from build123d import *

# Parameters (mm, degrees)
F0_R          = 12.5
F1_DEPTH      = 20
F1_DEPTH_BACK = 20
F3_DEPTH      = 40.001
F4_R          = 3
F5_DEPTH      = 25.001
F7_DEPTH      = 5


with BuildPart() as f1:
    # F0 (on Front) → F1 (new body, two sides)
    with BuildSketch(Plane.XZ) as f1_sk:
        with BuildLine():
            Line((49.364916731, 5), (19.364916731, 5))
            ThreePointArc((19.364916731, 5), (-20, 0), (19.364916731, -5))
            Line((19.364916731, -5), (49.364916731, -5))
            Line((49.364916731, -5), (49.364916731, 5))
        make_face()
        Circle(F0_R, mode=Mode.SUBTRACT)
    extrude(amount=F1_DEPTH)
    extrude(f1_sk.sketch, amount=-F1_DEPTH_BACK)

    # F2 (on face) → F3 (cut, through all)
    with BuildSketch(Plane.XZ.offset(20)):
        with BuildLine():
            Line((5.0842080384, 11.4193182205), (6.5077862892, 14.6167273223))
            ThreePointArc((6.5077862892, 14.6167273223), (4.6779472756, 15.3008760954), (2.7783708427, 15.7569240482))
            Line((2.7783708427, 15.7569240482), (2.1706022208, 12.3100969127))
            ThreePointArc((2.1706022208, 12.3100969127), (3.654646309, 11.9538094495), (5.0842080384, 11.4193182205))
        make_face()
        with BuildLine():
            Line((-3.8707503296, 15.5247316204), (-3.024023695, 12.1286965784))
            ThreePointArc((-3.024023695, 12.1286965784), (-1.5233667926, 12.4068268955), (0, 12.5))
            Line((0, 12.5), (0, 16))
            ThreePointArc((0, 16), (-1.9499094945, 15.8807384263), (-3.8707503296, 15.5247316204))
        make_face()
        with BuildLine():
            Line((-9.8505836052, 12.6081720577), (-7.6957684416, 9.8501344201))
            ThreePointArc((-7.6957684416, 9.8501344201), (-6.4379759364, 10.7145912588), (-5.0842080384, 11.4193182205))
            Line((-5.0842080384, 11.4193182205), (-6.5077862892, 14.6167273223))
            ThreePointArc((-6.5077862892, 14.6167273223), (-8.2406091986, 13.7146768112), (-9.8505836052, 12.6081720577))
        make_face()
        with BuildLine():
            Line((-14.1271614857, 7.5115450046), (-11.0368449107, 5.8683945348))
            ThreePointArc((-11.0368449107, 5.8683945348), (-10.2394005536, 7.1697054544), (-9.2893103185, 8.3641325795))
            Line((-9.2893103185, 8.3641325795), (-11.8903172076, 10.7060897017))
            ThreePointArc((-11.8903172076, 10.7060897017), (-13.1064327086, 9.1772229816), (-14.1271614857, 7.5115450046))
        make_face()
        with BuildLine():
            Line((-15.9610248042, 1.1161035799), (-12.4695506282, 0.8719559218))
            ThreePointArc((-12.4695506282, 0.8719559218), (-12.2703397931, 2.3851124422), (-11.8882064537, 3.8627124297))
            Line((-11.8882064537, 3.8627124297), (-15.2169042607, 4.94427191))
            ThreePointArc((-15.2169042607, 4.94427191), (-15.7060349352, 3.052943926), (-15.9610248042, 1.1161035799))
        make_face()
        with BuildLine():
            Line((-15.0350819326, -5.4723222932), (-11.7461577598, -4.2752517916))
            ThreePointArc((-11.7461577598, -4.2752517916), (-12.1796258098, -2.8118881793), (-12.4315236921, -1.3066057908))
            Line((-12.4315236921, -1.3066057908), (-15.9123503259, -1.6724554123))
            ThreePointArc((-15.9123503259, -1.6724554123), (-15.5899210366, -3.5992168695), (-15.0350819326, -5.4723222932))
        make_face()
        with BuildLine():
            Line((-11.5094368054, -11.1145339273), (-8.9917475042, -8.6832296307))
            ThreePointArc((-8.9917475042, -8.6832296307), (-9.9829438756, -7.5226877894), (-10.8253175473, -6.25))
            Line((-10.8253175473, -6.25), (-13.8564064606, -8))
            ThreePointArc((-13.8564064606, -8), (-12.7781681608, -9.6290403704), (-11.5094368054, -11.1145339273))
        make_face()
        with BuildLine():
            Line((-5.9937054947, -14.8349416731), (-4.6825824177, -11.5897981821))
            ThreePointArc((-4.6825824177, -11.5897981821), (-6.0601202531, -10.9327463392), (-7.3473156537, -10.1127124297))
            Line((-7.3473156537, -10.1127124297), (-9.4045640367, -12.94427191))
            ThreePointArc((-9.4045640367, -12.94427191), (-7.7569539239, -13.9939153142), (-5.9937054947, -14.8349416731))
        make_face()
        with BuildLine():
            Line((0.5583919472, -15.9902532323), (0.4362437088, -12.4923853377))
            ThreePointArc((0.4362437088, -12.4923853377), (-1.0894467843, -12.4524337261), (-2.5988961352, -12.2268450092))
            Line((-2.5988961352, -12.2268450092), (-3.3265870531, -15.6503616117))
            ThreePointArc((-3.3265870531, -15.6503616117), (-1.394491884, -15.9391151695), (0.5583919472, -15.9902532323))
        make_face()
        with BuildLine():
            Line((7.0139383486, -14.3807047408), (5.4796393349, -11.2349255787))
            ThreePointArc((5.4796393349, -11.2349255787), (4.0696019307, -11.818982195), (2.5988961352, -12.2268450092))
            Line((2.5988961352, -12.2268450092), (3.3265870531, -15.6503616117))
            ThreePointArc((3.3265870531, -15.6503616117), (5.2090904713, -15.1282972096), (7.0139383486, -14.3807047408))
        make_face()
        with BuildLine():
            Line((12.2567110899, -10.284601755), (9.575555539, -8.0348451211))
            ThreePointArc((9.575555539, -8.0348451211), (8.5249795008, -9.1419212702), (7.3473156537, -10.1127124297))
            Line((7.3473156537, -10.1127124297), (9.4045640367, -12.94427191))
            ThreePointArc((9.4045640367, -12.94427191), (10.911973761, -11.7016592259), (12.2567110899, -10.284601755))
        make_face()
        with BuildLine():
            Line((15.380187135, -4.4101976931), (12.0157711992, -3.4454669477))
            ThreePointArc((12.0157711992, -3.4454669477), (11.5063106682, -4.8841391061), (10.8253175473, -6.25))
            Line((10.8253175473, -6.25), (13.8564064606, -8))
            ThreePointArc((13.8564064606, -8), (14.7280776552, -6.2516980558), (15.380187135, -4.4101976931))
        make_face()
        with BuildLine():
            Line((15.8442890999, 2.2267696154), (12.3783508593, 1.739663762))
            ThreePointArc((12.3783508593, 1.739663762), (12.4980961895, 0.2181550805), (12.4315236921, -1.3066057908))
            Line((12.4315236921, -1.3066057908), (15.9123503259, -1.6724554123))
            ThreePointArc((15.9123503259, -1.6724554123), (15.9975631225, 0.279238503), (15.8442890999, 2.2267696154))
        make_face()
        with BuildLine():
            Line((13.5687695385, 8.4787082277), (10.600601202, 6.6239908029))
            ThreePointArc((10.600601202, 6.6239908029), (11.328847338, 5.2827282718), (11.8882064537, 3.8627124297))
            Line((11.8882064537, 3.8627124297), (15.2169042607, 4.94427191))
            ThreePointArc((15.2169042607, 4.94427191), (14.5009245926, 6.7618921879), (13.5687695385, 8.4787082277))
        make_face()
        with BuildLine():
            Line((8.9470864555, 13.2646011609), (6.9899112934, 10.3629696569))
            ThreePointArc((6.9899112934, 10.3629696569), (8.2007378624, 9.4338697528), (9.2893103185, 8.3641325795))
            Line((9.2893103185, 8.3641325795), (11.8903172076, 10.7060897017))
            ThreePointArc((11.8903172076, 10.7060897017), (10.4969444638, 12.0753532836), (8.9470864555, 13.2646011609))
        make_face()
    extrude(amount=-F3_DEPTH, mode=Mode.SUBTRACT)

    # F4 (on face) → F5 (cut, through all)
    with BuildSketch(Plane.XY.offset(5)):
        with Locations((26, 14)):
            Circle(F4_R)
        with Locations((42, 14)):
            Circle(F4_R)
        with Locations((26, -14)):
            Circle(F4_R)
        with Locations((42, -14)):
            Circle(F4_R)
    extrude(amount=-F5_DEPTH, mode=Mode.SUBTRACT)

    # F6 (on face) → F7 (cut)
    with BuildSketch(Plane(origin=(0, 0, -5), x_dir=(1, 0, 0), z_dir=(0, 0, -1))):
        Polygon((31.7735026919, 14), (28.8867513459, 19), (23.1132486541, 19), (20.2264973081, 14), (23.1132486541, 9), (28.8867513459, 9), align=None)
        Polygon((39.1132486541, 9), (44.8867513459, 9), (47.7735026919, 14), (44.8867513459, 19), (39.1132486541, 19), (36.2264973081, 14), align=None)
        Polygon((39.1132486541, -9), (36.2264973081, -14), (39.1132486541, -19), (44.8867513459, -19), (47.7735026919, -14), (44.8867513459, -9), align=None)
        Polygon((20.2264973081, -14), (23.1132486541, -19), (28.8867513459, -19), (31.7735026919, -14), (28.8867513459, -9), (23.1132486541, -9), align=None)
    extrude(amount=-F7_DEPTH, mode=Mode.SUBTRACT)


solid = f1.part
Geometry check sheet. Reference: the model listing, model coordinates, mm. A direction names the side the tool comes from. Round coordinates to 2 decimals unless told otherwise and drop trailing zeros. Order: outer loops, then holes, each group sorted by start corner. A loop starts at its lowest first (then second) coordinate and runs counter-clockwise, first axis right, second up. Notation, with made-up numbers: (70, 89.25) -> (122, 89.25) arc R30 ccw to (122, 127.25) -> close; hole circle Ø11 at (13.25, -0.75). An arc over 180 degrees is marked (long way). Use one line per item in the form item = value.
1. Go/stop test with flat-tipped pins: pin 1 (8 mm diameter, centred on x = 26, y = -14, fed in from +Z); pin 2 (3 mm diameter, centred on x = 41.5, y = -16, fed in from -Z); pin 3 (1 mm diameter, centred on x = 16, y = -9.5, fed in from +Z). Record where each tip stops, or that it passes through.
Working result:
pin_1 = 5
pin_2 = 0
pin_3 = 12.64
2. Cross-section at B-B, the plane x = 41.5. Enter the section's corners in (y, z), plus the area to 3 significant figures.
Working result:
outline = (-20, -5) -> (-19, -5) -> (-19, 0) -> (-16.96, 0) -> (-16.96, 5) -> (-20, 5) -> close; (-11.04, 0) -> (-9, 0) -> (-9, -5) -> (9, -5) -> (9, 0) -> (11.04, 0) -> (11.04, 5) -> (-11.04, 5) -> close; (16.96, 0) -> (19, 0) -> (19, -5) -> (20, -5) -> (20, 5) -> (16.96, 5) -> close
area = 241 mm^2
3. Set-up check for faces 4 (the face through (21.65, 16.465, -2.535)), 5 (the face through (34, 0, -5)), 6 (the face through (12.183, -0.28, 2.797)): record each of +Z, -Z, +X, -X, +Y, -Y from which the full face is reachable in a straight line by a thin tool's end or side.
Working result:
face_4 = -Z
face_5 = -Z, +X, +Y, -Y
face_6 = +Y, -Y
4. Scan lines: line 1 along Y through (x, z) = (26, 3.85); line 2 along X through (y, z) = (11, -9); line 3 along X through (y, z) = (1, -14.5). Record each from-to range of solid material in increasing order. Write a range as from..to.
Working result:
line_1 = -20..-17, -11..11, 17..20
line_2 = -17.86..-13.23, -9.32..-8.67, 10.73..17.86
line_3 = -13.77..-6.76, -5.86..-3.08, 0.51..3.08, 6.76..13.77
5. Mould release check, pull along X, two halves, no side actions. Record for faces 1 (the face through (-1.422, -0.28, -15.937)), 2 (the face through (35, 0, 5)), 3 (the face through (-19.984, -0.28, 0.809)): pulls with the +X half, pulls with the -X half, needs draft (parallel to the pull), parting line crosses it, or undercut.
Working result:
face_1 = undercut
face_2 = needs draft
face_3 = parting line crosses it
6. Cross-section at A-A, the plane x = 26. Enter the section's corners in (y, z), plus the area to 3 significant figures.
Working result:
outline = (-20, -5) -> (-19, -5) -> (-19, 0) -> (-17, 0) -> (-17, 5) -> (-20, 5) -> close; (-11, 0) -> (-9, 0) -> (-9, -5) -> (9, -5) -> (9, 0) -> (11, 0) -> (11, 5) -> (-11, 5) -> close; (17, 0) -> (19, 0) -> (19, -5) -> (20, -5) -> (20, 5) -> (17, 5) -> close
area = 240 mm^2
